from build123d import *

# Parameters (mm, degrees)
F0_R     = 6.1819299208
F1_DEPTH = 31.75
F3_DEPTH = 31.751
F2_W     = 15.875
F2_H     = 12.7
F2_W_2   = 9.525
F4_DEPTH = 31.751
F5_DEPTH = 31.751


with BuildPart() as f1:
    # F0 (on Top) → F1 (new body)
    with BuildSketch(Plane.XY):
        with BuildLine():
            Line((43.7930202991, -15.8396554504), (-48.2819797009, -15.8396554504))
            Line((-48.2819797009, -15.8396554504), (-48.2819797009, -25.3646554504))
            Line((-48.2819797009, -25.3646554504), (-7.0069797009, -25.3646554504))
            Line((-7.0069797009, -25.3646554504), (-7.0069797009, -38.0646554504))
            Line((-7.0069797009, -38.0646554504), (-48.2819797009, -38.0646554504))
            Line((-48.2819797009, -38.0646554504), (-48.2819797009, -47.5896554504))
            Line((-48.2819797009, -47.5896554504), (43.7930202991, -47.5896554504))
            ThreePointArc((43.7930202991, -47.5896554504), (59.6680202991, -31.7146554504), (43.7930202991, -15.8396554504))
        make_face()
        with Locations((43.7930202991, -31.7146554504)):
            Circle(F0_R, mode=Mode.SUBTRACT)
    extrude(amount=F1_DEPTH)

    # F2 (on face) → F3 (cut, through all)
    with BuildSketch(Plane.XZ.offset(47.5896554504)):
        with BuildLine():
            Line((-32.4069797009, 9.525), (-32.4069797009, 22.225))
            ThreePointArc((-32.4069797009, 22.225), (-38.7569797009, 15.875), (-32.4069797009, 9.525))
        make_face()
        with BuildLine():
            ThreePointArc((-26.0569797009, 15.875), (-27.9168516404, 20.3651280605), (-32.4069797009, 22.225))
            Line((-32.4069797009, 22.225), (-32.4069797009, 9.525))
            ThreePointArc((-32.4069797009, 9.525), (-27.9168516404, 11.3848719395), (-26.0569797009, 15.875))
        make_face()
    extrude(amount=-F3_DEPTH, mode=Mode.SUBTRACT)

    # F2 (on face) → F4 (cut, through all)
    with BuildSketch(Plane.XZ.offset(47.5896554504)):
        with Locations((51.7305202991, 15.875)):
            Rectangle(F2_W, F2_H)
        with Locations((39.0305202991, 15.875)):
            Rectangle(F2_W_2, F2_H)
    extrude(amount=-F4_DEPTH, mode=Mode.SUBTRACT)

    # F2 (on face) → F5 (cut, through all)
    with BuildSketch(Plane.XZ.offset(47.5896554504)):
        with BuildLine():
            ThreePointArc((-48.2819797009, 15.875), (-43.6322998523, 27.1003201513), (-32.4069797009, 31.75))
            Line((-32.4069797009, 31.75), (-48.2819797009, 31.75))
            Line((-48.2819797009, 31.75), (-48.2819797009, 15.875))
        make_face()
        with BuildLine():
            ThreePointArc((-32.4069797009, 0), (-43.6322998523, 4.6496798487), (-48.2819797009, 15.875))
            Line((-48.2819797009, 15.875), (-48.2819797009, 0))
            Line((-48.2819797009, 0), (-32.4069797009, 0))
        make_face()
    extrude(amount=-F5_DEPTH, mode=Mode.SUBTRACT)


solid = f1.part
Check sheet for the modelled part. Datum: model origin and axes. Units: mm. A direction names the side the tool comes from. Round coordinates to 2 decimals unless told otherwise and drop trailing zeros. Loops run counter-clockwise (first coordinate to the right, second up) from the corner with the lowest first, then second, coordinate; pieces in that order, holes last.
1. Set-up check for faces 4 (the flat face through (34.268, -32, 16)), 5 (the flat face through (-7.007, -32, 16)), 6 (the flat face through (13, -31, 31.75)): record each of +Z, -Z, +X, -X, +Y, -Y from which the full face is reachable in a straight line by a thin tool's end or side.
2. Sectioned sample at B-B on x = -29.5. Record the boundary of the cut face in (y, z), and give its area (3 significant figures).
3. Gauge pin test, flat ends, axial feed: pin 1 Ø5 at (y, z) = (-36.5, 9) entering from -X; pin 2 Ø3 at (y, z) = (-24, 27.5) entering from -X; pin 3 Ø7.5 at (x, y) = (43.79, -31.71) entering from +Z; pin 4 Ø12 at (y, z) = (-22.5, 16) entering from +X. Record the tip position at first contact, or that the pin passes through.
4. Sectioned sample at D-D on y = -19.5. Record the boundary of the cut face in (x, z) (3 decimals), and give its area (3 significant figures).
5. Sectioned sample at C-C on z = 24. Record the boundary of the cut face in (x, y) (3 decimals), and give its area (3 significant figures).
6. Sectioned sample at A-A on y = -33. Record the boundary of the cut face in (x, z) (3 decimals), and give its area (3 significant figures).
7. Scan lines: probe 1 along Y at (x, z) = (-9, 5); probe 2 along Z at (x, y) = (50, -19.5) (3 decimals); probe 3 along X at (y, z) = (-33, 6). Record each from-to range of solid material in increasing order.
8. Mould release check, pull along Z, two halves, no side actions. Record for faces 1 (the flat face through (-23, -38.065, 16)), 2 (the flat face through (13, -31, 0)), 3 (the flat face through (50, -28, 22.225)): released by +Z, released by -Z, zero draft, split by the parting line, or undercut.
Recorded:
1. face 4: +X, +Y, -Y
1. face 5: +Z, -Z, -X
1. face 6: +Z, +X, -X, +Y, -Y
2. outline: (-47.59, 0) - (-38.06, 0) - (-38.06, 10.23) - (-47.59, 10.23) - close; (-47.59, 21.52) - (-38.06, 21.52) - (-38.06, 31.75) - (-47.59, 31.75) - close; (-25.36, 0) - (-15.84, 0) - (-15.84, 10.23) - (-25.36, 10.23) - close; (-25.36, 21.52) - (-15.84, 21.52) - (-15.84, 31.75) - (-25.36, 31.75) - close
2. area: 390 mm2
3. pin 1: stops at x = -47.5
3. pin 2: stops at x = -44.63
3. pin 3: passes through
3. pin 4: stops at x = 34.27
4. outline: (-32.407, 0) - (53.933, 0) - (53.933, 9.525) - (34.268, 9.525) - (34.268, 22.225) - (53.933, 22.225) - (53.933, 31.75) - (-32.407, 31.75) arc R15.875 ccw to start; hole circle Ø12.7 at (-32.407, 15.875)
4. area: 2,760 mm2
5. outline: (-46.045, -47.59) - (43.793, -47.59) arc R15.875 ccw to (43.793, -15.84) - (-46.045, -15.84) - (-46.045, -25.365) - (-7.007, -25.365) - (-7.007, -38.065) - (-46.045, -38.065) - close; hole circle Ø12.364 at (43.793, -31.715)
5. area: 2,630 mm2
6. outline: (-7.007, 0) - (37.746, 0) - (37.746, 9.525) - (34.268, 9.525) - (34.268, 22.225) - (37.746, 22.225) - (37.746, 31.75) - (-7.007, 31.75) - close; (49.84, 0) - (59.616, 0) - (59.616, 9.525) - (49.84, 9.525) - close; (49.84, 22.225) - (59.616, 22.225) - (59.616, 31.75) - (49.84, 31.75) - close
6. area: 1,560 mm2
7. probe 1: y = -47.59 to -38.06, -25.36 to -15.84
7. probe 2: z = 0 to 9.525, 22.225 to 31.75
7. probe 3: x = -7.01 to 37.75, 49.84 to 59.62
8. face 1: zero draft
8. face 2: released by -Z
8. face 3: undercut
